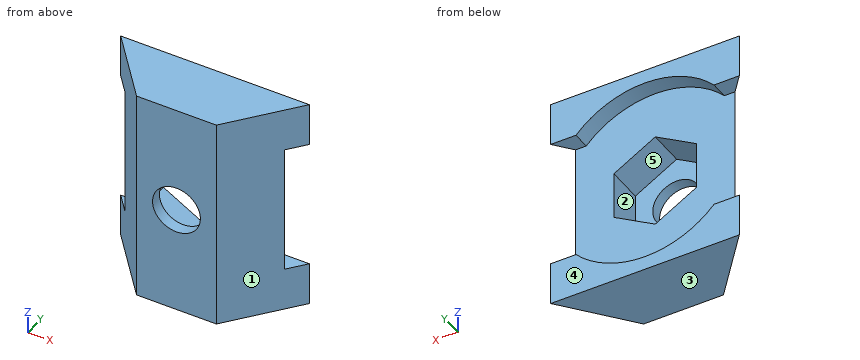
```python
from build123d import *

# Parameters (mm, degrees)
RESSALTO_EXTRUS_O1_DEPTH = 15
ESBO_O2_R                = 1.65
CORTE_EXTRUS_O1_DEPTH    = 15
CORTE_EXTRUS_O5_DEPTH    = 1.2
CORTE_EXTRUS_O6_DEPTH    = 2.5


with BuildPart() as part:
    # Esboço1 → Ressalto-extrusão1 (new body)
    with BuildSketch(Plane.XY):
        Polygon((-6.5, 0), (6.5, 0), (2.75, -4.5), (-2.75, -4.5), align=None)
    extrude(amount=RESSALTO_EXTRUS_O1_DEPTH)

    # Esboço2 → Corte-extrusão1 (cut)
    with BuildSketch(Plane(origin=(0, 0, 0), x_dir=(1, 0, 0), z_dir=(0, 1, 0))):
        with Locations((0, -7.5)):
            Circle(ESBO_O2_R)
    extrude(amount=-CORTE_EXTRUS_O1_DEPTH, mode=Mode.SUBTRACT)

    # Esboço3 → Corte-extrusão5 (cut)
    with BuildSketch(Plane(origin=(0, 0, 0), x_dir=(1, 0, 0), z_dir=(0, 1, 0))):
        with BuildLine():
            Line((4.759464256, -3), (7.813565265, -3))
            Line((7.813565265, -3), (7.813565265, -12))
            Line((7.813565265, -12), (4.759464256, -12))
            ThreePointArc((4.759464256, -12), (0, -14.05), (-4.759464256, -12))
            Line((-4.759464256, -12), (-7.813565265, -12))
            Line((-7.813565265, -12), (-7.813565265, -3))
            Line((-7.813565265, -3), (-4.759464256, -3))
            ThreePointArc((-4.759464256, -3), (0, -0.95), (4.759464256, -3))
        make_face()
    extrude(amount=-CORTE_EXTRUS_O5_DEPTH, mode=Mode.SUBTRACT)

    # Esboço4 → Corte-extrusão6 (cut)
    with BuildSketch(Plane(origin=(0, -1.2, 0), x_dir=(1, 0, 0), z_dir=(0, 1, 0))):
        Polygon((0, -4.209103466), (-2.85, -5.854551733), (-2.85, -9.145448267), (0, -10.790896534), (2.85, -9.145448267), (2.85, -5.854551733), align=None)
    extrude(amount=-CORTE_EXTRUS_O6_DEPTH, mode=Mode.SUBTRACT)


solid = part.part
```
Can you work these out from the model? Positions are in its coordinate system, mm. Face numbers are marked on the shaded views. A direction names the side the tool comes from. Coordinates: 2 decimals unless noted, no trailing zeros. Write each loop counter-clockwise with the first axis right and the second up, starting at its lowest first coordinate (ties: lowest second). Pieces come first, ordered by that corner, then holes. Notation, with made-up numbers: (45.5, 77) - (95.5, 77) arc R12 ccw to (95.5, 90) - close; hole circle Ø11 at (-16.75, 54.25). An arc over 180 degrees is marked (long way). Return JSON: item names as keys, results as strings.
Q1. If we section it at C-C (x = -1): Please give me the cut outline in (y, z), then the cut area to 3 significant figures.
Computed values:
{"outline": "(-4.5, 0) - (0, 0) - (0, 1.03) - (-1.2, 1.03) - (-1.2, 4.79) - (-3.7, 4.79) - (-3.7, 6.19) - (-4.5, 6.19) - close; (-4.5, 8.81) - (-3.7, 8.81) - (-3.7, 10.21) - (-1.2, 10.21) - (-1.2, 13.97) - (0, 13.97) - (0, 15) - (-4.5, 15) - close", "area": "36.3 mm2"}
Q2. Thinking about a two-plate mould opening in X: for the marked faces 1, 2 and 3, which applies, +X half, -X half, draft (parallel to the pull), parting line (faces both ways), or undercut?
Computed values:
{"face 1": "+X half", "face 2": "undercut", "face 3": "draft"}
Q3. If we section it at A-A (z = 7.5): Please give me the cut outline in (x, y), then the cut area to 3 significant figures.
Computed values:
{"outline": "(-5.5, -1.2) - (-2.75, -4.5) - (-1.65, -4.5) - (-1.65, -3.7) - (-2.85, -3.7) - (-2.85, -1.2) - close; (1.65, -4.5) - (2.75, -4.5) - (5.5, -1.2) - (2.85, -1.2) - (2.85, -3.7) - (1.65, -3.7) - close", "area": "10.3 mm2"}
Q4. If we section it at B-B (y = -0.6): Please give me the cut outline in (x, z).
Computed values:
{"outline": "(-6, 0) - (6, 0) - (6, 3) - (4.76, 3) arc R6.55 cw to (-4.76, 3) - (-6, 3) - close; (-6, 12) - (-4.76, 12) arc R6.55 cw to (4.76, 12) - (6, 12) - (6, 15) - (-6, 15) - close"}
Q5. I'm going to push flat-ended pins straight in: pin 1 Ø4 at (x, z) = (-1.5, 8) entering from +Y; pin 2 Ø0.8 at (y, z) = (-2.5, 7.5) entering from +X; pin 3 Ø4.5 at (x, z) = (0, 7.5) entering from +Y. Where does each tip first touch, or does it pass through?
Computed values:
{"pin 1": "stops at y = -1.2", "pin 2": "stops at x = 4.75", "pin 3": "stops at y = -3.7"}
Q6. If we section it at D-D (y = -2.5): Please give me the cut outline in (x, z).
Computed values:
{"outline": "(-4.42, 0) - (4.42, 0) - (4.42, 15) - (-4.42, 15) - close; hole (-2.85, 5.85) - (0, 4.21) - (2.85, 5.85) - (2.85, 9.15) - (0, 10.79) - (-2.85, 9.15) - close"}
Q7. On a 3-axis mill with a long thin cutter (end or side, diameter ignored), from which of +Z, -Z, +X, -X, +Y, -Y can I reach the whole of each face in a straight line? I mean the marked faces 4 and 5. Say none if no direction works.
Computed values:
{"face 4": "+Z, -Z, +X, -X, +Y", "face 5": "+Y"}
Q8. Please list where these lines run through material, in increasing order: L1, parallel to Z at x = -5, y = -0.6; L2, parallel to Z at x = 0, y = -4.2; L3, parallel to X at y = -3.9, z = 7.5. Write a range as from..to.
Computed values:
{"L1": "z = 0..3, 12..15", "L2": "z = 0..5.85, 9.15..15", "L3": "x = -3.25..-1.65, 1.65..3.25"}
